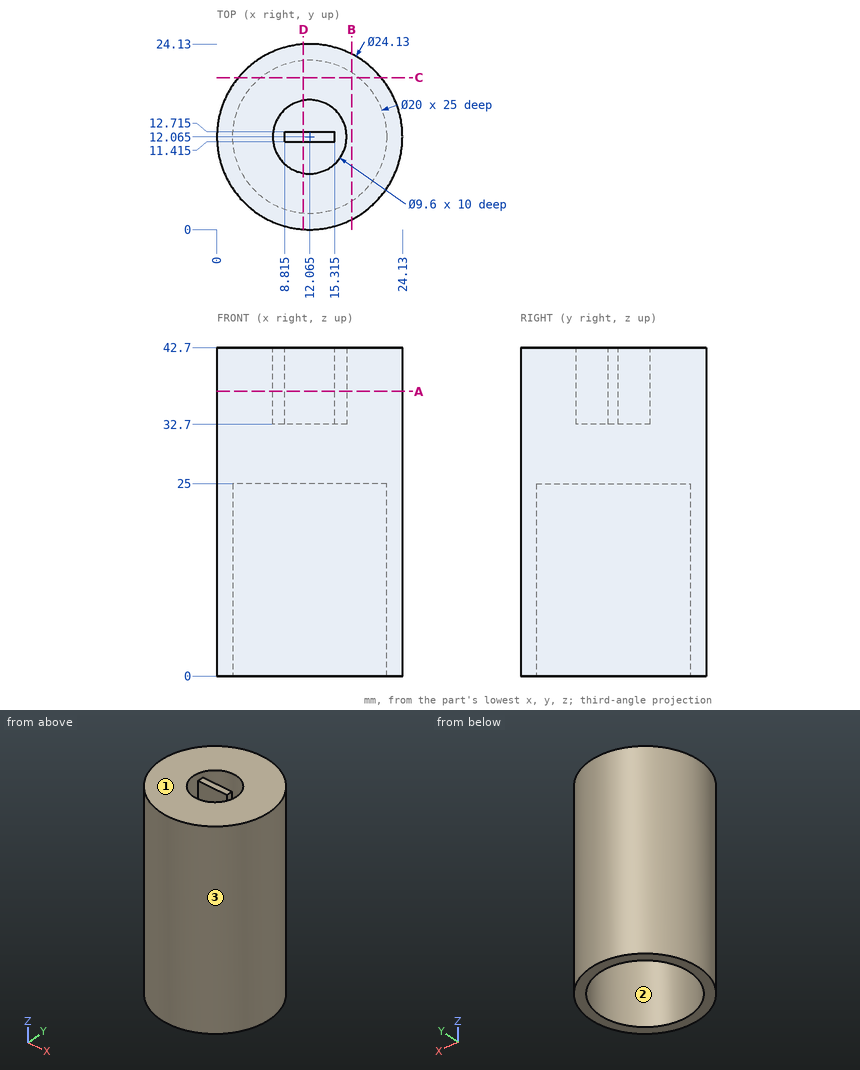
Source: three-view drawing plus pictorial views. Frame: mm from the lowest corner of the part. Coordinates: 2 decimals unless noted, no trailing zeros. Write each loop counter-clockwise with the first axis right and the second up, starting at its lowest first coordinate (ties: lowest second). Pieces come first, ordered by that corner, then holes. Notation, with made-up numbers: (45, 6) - (59, 6) arc R17 ccw to (59, 22) - close; hole circle Ø2 at (-11.75, -6). An arc over 180 degrees is marked (long way). Return JSON: item names as keys, results as strings.
Item 1: Pin query (flat end, axial travel): pin 1 Ø10 at (x, y) = (17, 12) entering from -Z; pin 2 Ø12 at (y, z) = (4.5, 19.5) entering from -X; pin 3 Ø1 at (y, z) = (6, 6.5) entering from -X. Return the tip coordinate at first contact, or that it passes through.
Completed:
{"pin 1": "stops at z = 25", "pin 2": "stops at x = 0.1", "pin 3": "stops at x = 1.36"}
Item 2: Section query B-B (x = 17.5). Output: boundary loops of the cut face in (y, z).
Completed:
{"outline": "(1.29, 0) - (3.67, 0) - (3.67, 25) - (20.46, 25) - (20.46, 0) - (22.84, 0) - (22.84, 42.7) - (1.29, 42.7) - close"}
Item 3: Pull-direction query (X, two-part tool) for the marked faces 1, 2 and 3; classes: +X half, -X half, draft (parallel to the pull), parting line (faces both ways), or undercut.
Completed:
{"face 1": "draft", "face 2": "undercut", "face 3": "parting line"}
Item 4: Line query: L1, parallel to Y at x = 12.5, z = 5; L2, parallel to Y at x = 13, z = 39 (3 decimals); L3, parallel to Z at x = 18.5, y = 7.5. Output: solid intervals per line, ascending.
Completed:
{"L1": "y = 0.01 to 2.07, 22.06 to 24.12", "L2": "y = 0.036 to 7.357, 11.415 to 12.715, 16.773 to 24.094", "L3": "z = 25 to 42.7"}
Item 5: Section query A-A (z = 37). Output: boundary loops of the cut face in (x, y) (3 decimals).
Completed:
{"outline": "circle Ø24.13 at (12.065, 12.065); (8.815, 11.415) - (15.315, 11.415) - (15.315, 12.715) - (8.815, 12.715) - close; hole circle Ø9.6 at (12.065, 12.065)"}
Item 6: Section query D-D (x = 11.25). Output: boundary loops of the cut face in (y, z) (3 decimals).
Completed:
{"outline": "(0.028, 0) - (2.098, 0) - (2.098, 25) - (22.032, 25) - (22.032, 0) - (24.102, 0) - (24.102, 42.7) - (16.795, 42.7) - (16.795, 32.7) - (12.715, 32.7) - (12.715, 42.7) - (11.415, 42.7) - (11.415, 32.7) - (7.335, 32.7) - (7.335, 42.7) - (0.028, 42.7) - close"}
Item 7: Section query C-C (y = 19.75). Output: boundary loops of the cut face in (x, z).
Completed:
{"outline": "(2.76, 0) - (5.67, 0) - (5.67, 25) - (18.46, 25) - (18.46, 0) - (21.37, 0) - (21.37, 42.7) - (2.76, 42.7) - close"}
